CAD build for the part. Positions are in the model's coordinates, mm. A direction names the side the tool comes from. Coordinates: 2 decimals unless noted, no trailing zeros. Order: outer loops, then holes, each group sorted by start corner. A loop starts at its lowest first (then second) coordinate and runs counter-clockwise, first axis right, second up. Notation, with made-up numbers: (78.5, 59.5) - (103.5, 59.5) arc R12 ccw to (103.5, 65.5) - close; hole circle Ø8 at (-22, -28.5). An arc over 180 degrees is marked (long way). Return JSON: item names as keys, results as strings.
from build123d import *
from build123d import SkipClean  # not in build123d's __all__

# Parameters (mm, degrees)
F1_DEPTH  = 14.5
F3_DEPTH  = 20
F5_DEPTH  = 5
F7_DEPTH  = 5
F9_DEPTH  = 2.5
F10_DEPTH = 15
F12_DEPTH = 2.5
F14_SIZE  = 2.49999
F16_DEPTH = 15
F18_DEPTH = 2.5
F22_R     = 20
F23_DEPTH = 2.5
F24_SIZE  = 2.49999
F25_R     = 10
F26_DEPTH = 17.001
F27_R     = 10
F28_DEPTH = 17.001
F29_R     = 10
F30_DEPTH = 135.001
F31_R     = 10
F32_DEPTH = 75.501
F33_R     = 10
F34_DEPTH = 90.001
F35_R     = 2.5


# Not quite as in the source:
# - a fillet or chamfer that OpenCascade refuses, or shapes differently, is made with other operations: its cross-section is extruded or revolved along the edge and cut away or added
# - a fillet or chamfer is up to 0.001 mm smaller than in the source, because OpenCascade refuses the exact size
# - a feature of the source that left no trace in its solid (it failed there, or was rolled back) is left out
# - a pattern or mirror of a feature is missing from the dataset's text; its kind, count and spacing are read off the source's solid


with BuildPart() as f1:
    # F0 (on Top) → F1 (new body)
    with BuildSketch(Plane.XY):
        with BuildLine():
            ThreePointArc((25, 70), (0, 95), (-25, 70))
            Line((-25, 70), (-25, -70))
            ThreePointArc((-25, -70), (0, -95), (25, -70))
            Line((25, -70), (25, -25))
            Line((25, -25), (75, -25))
            ThreePointArc((75, -25), (100, 0), (75, 25))
            Line((75, 25), (25, 25))
            Line((25, 25), (25, 70))
        make_face()
    extrude(amount=F1_DEPTH)

    # F2 (on Right) → F3 (join, symmetric)
    with BuildSketch(Plane.YZ):
        Polygon((-37.5, 70), (-37.5, 0), (37.5, 0), (37.5, 70), (22.5, 70), (22.5, 27), (-22.5, 27), (-22.5, 70), align=None)
    extrude(amount=F3_DEPTH, both=True)

    # F4 (on Right) → F5 (join, symmetric)
    with BuildSketch(Plane.YZ):
        Polygon((-37.5, 49.5), (-49.5, 14.5), (-37.5, 14.5), align=None)
        Polygon((37.5, 49.5), (37.5, 14.5), (49.5, 14.5), align=None)
    extrude(amount=F5_DEPTH, both=True)

    # F6 (on Front) → F7 (join, symmetric)
    with BuildSketch(Plane.XZ):
        Polygon((26, 27), (20, 27), (20, 14.5), (54, 14.5), align=None)
    extrude(amount=F7_DEPTH, both=True)

    # F8 (on face) → F9 (join)
    with BuildSketch(Plane.XZ.offset(37.5)):
        with BuildLine():
            ThreePointArc((-20, 70), (0, 50), (20, 70))
            Line((20, 70), (-20, 70))
        make_face()
        with BuildLine():
            Line((-20, 70), (20, 70))
            ThreePointArc((20, 70), (0, 90), (-20, 70))
        make_face()
    extrude(amount=F9_DEPTH)

    # F10 (add): a face of the model
    f10_faces = [f1.faces().sort_by_distance(p)[0] for p in [
        (0, -37.5, 78.4882636316),
    ]]
    extrude(f10_faces, amount=F10_DEPTH)

    # F11 (on face) → F12 (join)
    with BuildSketch(Plane(origin=(0, -22.5, 0), x_dir=(-1, 0, 0), z_dir=(0, 1, 0))):
        with BuildLine():
            ThreePointArc((-20, 70), (0, 50), (20, 70))
            ThreePointArc((20, 70), (0, 90), (-20, 70))
        make_face()
    f12 = extrude(amount=F12_DEPTH)

    # F12_copies: F12 across plane
    add(f12.mirror(Plane.ZX), clean=False)

    # F13: chamfer of 2.5 on 1 edges, made by hand

    # F13_s1 → F13_t2 (revolve, cut)
    with BuildSketch(Plane.XY.offset(70)):
        Polygon((20, -22.5), (17.5, -20), (20, -20), align=None)
    revolve(axis=Axis((0, -20, 70), (0, -1, 0)), mode=Mode.SUBTRACT)

    # F14 (size 2.5 in the source; OpenCascade refuses exactly that, so slightly less here)
    f14_edges = [f1.edges().sort_by_distance(p)[0] for p in [
        (-20, -40, 70),
    ]]
    chamfer(f14_edges, length=F14_SIZE)

    # F15 (on face) → F16 (join)
    with BuildSketch(Plane(origin=(0, 37.5, 0), x_dir=(-1, 0, 0), z_dir=(0, 1, 0))):
        with BuildLine():
            ThreePointArc((-20, 70), (0, 50), (20, 70))
            Line((20, 70), (-20, 70))
        make_face()
        with BuildLine():
            Line((-20, 70), (20, 70))
            ThreePointArc((20, 70), (0, 90), (-20, 70))
        make_face()
    extrude(amount=-F16_DEPTH)

    # F17 (on face) → F18 (join)
    with BuildSketch(Plane(origin=(0, 37.5, 0), x_dir=(-1, 0, 0), z_dir=(0, 1, 0))):
        with BuildLine():
            ThreePointArc((-20, 70), (0, 50), (20, 70))
            ThreePointArc((20, 70), (0, 90), (-20, 70))
        make_face()
    with SkipClean():  # cleaning this boolean's faces spoils the solid; the shape is the same uncleaned
        extrude(amount=F18_DEPTH)

    # F21: chamfer of 2.5 on 2 edges, made by hand

    # F21_s1 → F21_t2 (revolve, cut)
    with BuildSketch(Plane.XY.offset(70)):
        Polygon((20, 37.5), (17.5, 40), (20, 40), align=None)
    revolve(axis=Axis((0, 40, 70), (0, -1, 0)), mode=Mode.SUBTRACT)

    # F21_s3 → F21_t4 (revolve, cut)
    with BuildSketch(Plane.XY.offset(70)):
        Polygon((20, 22.5), (17.5, 20), (20, 20), align=None)
    revolve(axis=Axis((0, 20, 70), (0, -1, 0)), mode=Mode.SUBTRACT)

    # F22 (on face) → F23 (join)
    with BuildSketch(Plane.XY.offset(14.5)):
        with Locations((0, 70)):
            Circle(F22_R)
        with Locations((75, 0)):
            Circle(F22_R)
        with Locations((0, -70)):
            Circle(F22_R)
    extrude(amount=F23_DEPTH)

    # F24 (size 2.5 in the source; OpenCascade refuses exactly that, so slightly less here)
    f24_edges = [f1.edges().sort_by_distance(p)[0] for p in [
        (-20, 70, 17),
        (55, 0, 17),
        (-20, -70, 17),
    ]]
    chamfer(f24_edges, length=F24_SIZE)

    # F25 (on face) → F26 (cut, through all)
    with BuildSketch(Plane.XY.offset(17)):
        with Locations((0, 70)):
            Circle(F25_R)
    extrude(amount=-F26_DEPTH, mode=Mode.SUBTRACT)

    # F27 (on face) → F28 (cut, through all)
    with BuildSketch(Plane.XY.offset(17)):
        with Locations((75, 0)):
            Circle(F27_R)
    extrude(amount=-F28_DEPTH, mode=Mode.SUBTRACT)

    # F29 (on face) → F30 (cut, through all)
    with BuildSketch(Plane.XZ.offset(40)):
        with Locations((0, 70)):
            Circle(F29_R)
    extrude(amount=-F30_DEPTH, mode=Mode.SUBTRACT)

    # F31 (on face) → F32 (cut, through all)
    with BuildSketch(Plane.XY.offset(14.5)):
        with Locations((0, -70)):
            Circle(F31_R)
    extrude(amount=F32_DEPTH, mode=Mode.SUBTRACT)

    # F33 (on face) → F34 (cut, through all)
    with BuildSketch(Plane(origin=(0, 0, 0), x_dir=(1, 0, 0), z_dir=(0, 0, -1))):
        with Locations((0, 70)):
            Circle(F33_R)
    extrude(amount=-F34_DEPTH, mode=Mode.SUBTRACT)

    # F35
    f35_edges = [f1.edges().sort_by_distance(p)[0] for p in [
        (0, 22.5, 27),
        (0, -22.5, 27),
        (25, 25, 7.25),
        (25, -25, 7.25),
    ]]
    fillet(f35_edges, radius=F35_R)


solid = f1.part
Item 1: Wall check: L1, parallel to Y at x = 0, z = 9; L2, parallel to Y at x = 75, z = 8; L3, parallel to Y at x = -12, z = 65. Give the ranges that are in metal, low to high. Write a range as [from, to].
Findings below:
{"L1": "y = [-95, -80], [-60, 60], [80, 95]", "L2": "y = [-25, -10], [10, 25]", "L3": "y = [-40, -20], [20, 40]"}
Item 2: Band-saw the part on B-B, the plane z = 46.5. List the corners of the cut face in (x, y).
Findings below:
{"outline": "(-20, -37.5) - (-5, -37.5) - (-5, -38.53) - (5, -38.53) - (5, -37.5) - (20, -37.5) - (20, -22.5) - (-20, -22.5) - close; (-20, 22.5) - (20, 22.5) - (20, 37.5) - (5, 37.5) - (5, 38.53) - (-5, 38.53) - (-5, 37.5) - (-20, 37.5) - close"}
Item 3: Drop flat-ended pins along their axis: P1, Ø1, axis at x = 6, z = 37.5, coming from the -Y side; P2, Ø13, axis at y = 45.5, z = 36.5, coming from the +X side; P3, Ø9.5, axis at y = 44.5, z = 36, coming from the -X side; P4, Ø18, axis at x = 75, y = 0, coming from the -Z side. Give the stop position or say it passes through.
Findings below:
{"P1": "stops at y = -37.5", "P2": "stops at x = 5", "P3": "stops at x = -5", "P4": "passes through"}
Item 4: Band-saw the part on D-D, the plane x = 0. Count the separate pieces of the cut face and the enclosed holes in it, then the cut area to 3 significant figures.
Findings below:
{"separate pieces": "5", "enclosed holes": "0", "area": "5,090 mm²"}
Item 5: Which spindle directions (+Z, -Z, +X, -X, +Y, -Y) get a long thin tool onto all of the face, cutting with end or side? Do faces 4 (the flat face through (52, 25, 7)), 5 (the flat face through (8, -40, 62)), 6 (the flat face through (3, 0, 27)), 7 (the flat face through (-5, 41, 24)). Say none if no direction does.
Findings below:
{"face 4": "+Z, -Z, +X, +Y", "face 5": "+Z, +X, -X, -Y", "face 6": "+Z, +X, -X", "face 7": "-X"}
Item 6: Band-saw the part on C-C, the plane y = -32. List the corners of the cut face in (x, z), then the cut area to 3 significant figures.
Findings below:
{"outline": "(-25, 0) - (25, 0) - (25, 14.5) - (20, 14.5) - (20, 70) arc R20 ccw to (-20, 70) - (-20, 14.5) - (-25, 14.5) - close; hole circle Ø20 at (0, 70)", "area": "3,260 mm²"}
Item 7: Mould opens along Y. For faces 1 (the flat face through (23, 1, 0)), 2 (the conical face through (9.47, -39.88, 84.86)), 3 (the flat face through (0, -22.5, 40)) say: released by +Y, released by -Y, zero draft, split by the parting line, or undercut.
Findings below:
{"face 1": "zero draft", "face 2": "released by -Y", "face 3": "undercut"}
